```python
from build123d import *

# Parameters (mm, degrees)
BOSS_EXTRUDE1_DEPTH     = 101.6
CUT_EXTRUDE2_DEPTH      = 77.2
CUT_EXTRUDE2_DEPTH_BACK = 51.8
CUT_EXTRUDE6_DEPTH      = 50.8


with BuildPart() as part:
    # Sketch1 → Boss-Extrude1 (new body)
    with BuildSketch(Plane.XY):
        Polygon((-63.5, 76.2), (-12.7, 76.2), (-12.7, 25.4), (63.5, 25.4), (63.5, 0), (-63.5, 0), align=None)
    extrude(amount=BOSS_EXTRUDE1_DEPTH)

    # Sketch2 → Cut-Extrude2 (cut, two sides)
    with BuildSketch(Plane(origin=(-12.7, 0, 0), x_dir=(0, 0, -1), z_dir=(1, 0, 0))) as cut_extrude2_sk:
        Polygon((236.128778424, 194.264389212), (0, 76.2), (-101.6, 25.4), (-337.728778424, -92.664389212), (-573.857556848, 379.593167636), (0, 666.52194606), align=None)
    extrude(amount=CUT_EXTRUDE2_DEPTH, mode=Mode.SUBTRACT)
    extrude(cut_extrude2_sk.sketch, amount=-CUT_EXTRUDE2_DEPTH_BACK, mode=Mode.SUBTRACT)

    # Sketch3 → Cut-Extrude6 (cut)
    with BuildSketch(Plane.XY.offset(101.6)):
        Polygon((63.5, 25.4), (12.7, 25.4), (63.5, 0), align=None)
    extrude(amount=-CUT_EXTRUDE6_DEPTH, mode=Mode.SUBTRACT)


solid = part.part
```
Source: CAD feature listing. Evaluate the final solid. Frame: model axes, mm. A direction names the side the tool comes from. Give positions to 0.01 mm unless a question says otherwise; leave off trailing zeros. Order: outer loops, then holes, each group sorted by start corner. A loop starts at its lowest first (then second) coordinate and runs counter-clockwise, first axis right, second up.
(1) Contact query for flat-ended pins moving along their axis: P1, Ø1.5, axis at x = -27, y = 58, coming from the +Z side; P2, Ø1.5, axis at x = -14, y = 65.5, coming from the +Z side; P3, Ø8, axis at y = 9.5, z = 80.5, coming from the +X side. Output: stop coordinate, or through.
(2) Material intervals for line 1 along Y through (x, z) = (15.5, 14.5); line 2 along X through (y, z) = (49.5, 35.5); line 3 along Y through (x, z) = (-27.5, 19), sorted ascending.
(3) Access query for faces 1 (the face through (49, 19, 50.8)), 2 (the face through (-13, 13, 101.6)), 3 (the face through (16, 25.4, 39)). Directions: +Z, -Z, +X, -X, +Y, -Y. A direction counts if a zero-diameter tool reaches every point of the face in a straight line with its end or side. Return the directions, or none.
(4) Section query B-B (z = 68). Return the cut outline in (x, y).
(5) Section query C-C (x = -3). Return the cut outline in (y, z), plus the area to 3 significant figures.
(6) Section query A-A (y = 7). Return the cut outline in (x, z).
(7) Section query D-D (y = 66.5). Return the cut outline in (x, z).
Outcome:
1. P1: stops at z = 37.9
1. P2: stops at z = 22.9
1. P3: stops at x = 52.5
2. line 1: y = 0 to 25.4
2. line 2: x = -63.5 to -12.7
2. line 3: y = 0 to 66.7
3. face 1: +Z, +X, +Y
3. face 2: +Z, +X, -X, +Y, -Y
3. face 3: +Z, -Z, +X, +Y
4. outline: (-63.5, 0) - (63.5, 0) - (12.7, 25.4) - (-12.7, 25.4) - (-12.7, 42.2) - (-63.5, 42.2) - close
5. outline: (0, 0) - (25.4, 0) - (25.4, 101.6) - (0, 101.6) - close
5. area: 2,580 mm2
6. outline: (-63.5, 0) - (63.5, 0) - (63.5, 50.8) - (49.5, 50.8) - (49.5, 101.6) - (-63.5, 101.6) - close
7. outline: (-63.5, 0) - (-12.7, 0) - (-12.7, 19.4) - (-63.5, 19.4) - close
